Verification items for the finished model (mm, model axes). A direction names the side the tool comes from. Coordinates: 2 decimals unless noted, no trailing zeros. Write each loop counter-clockwise with the first axis right and the second up, starting at its lowest first coordinate (ties: lowest second). Pieces come first, ordered by that corner, then holes. Notation, with made-up numbers: (-17.75, 23.5) - (-2.75, 23.5) arc R22 cw to (-2.75, 59.5) - close; hole circle Ø8 at (-25, 10). An arc over 180 degrees is marked (long way). Use one line per item in the form item = value. Start each with the question number.
(1) Material ranges on line 1 (Y direction, x = -1, z = -2); line 2 (Y direction, x = 2, z = 1.75); line 3 (Y direction, x = -3.5, z = 4), recorded low to high. Write a range as [from, to].
(2) Gauge pin test, flat ends, axial feed: pin 1 Ø1 at (x, z) = (1.5, -3) entering from +Y; pin 2 Ø6 at (x, y) = (-3.5, 3) entering from +Z; pin 3 Ø3 at (y, z) = (8.5, -0.5) entering from -X; pin 4 Ø3 at (y, z) = (12, -4.5) entering from +X. Record the tip position at first contact, or that the pin passes through.
(3) Sectioned sample at D-D (y = 8.25). Record the cut outline in (x, z).
(4) Sectioned sample at C-C (y = 2). Record the cut outline in (x, z), and give its area (3 significant figures).
(5) Tool access check on faces 1 (the flat face through (-1.8, 5.6, 3)), 2 (the flat face through (-3.5, 6, 0)), 3 (the flat face through (3.5, 6, 0)). Record the directions out of +Z, -Z, +X, -X, +Y, -Y that give a thin tool (end or side, any length) a straight path to the whole face; none if there is none.
(6) Sectioned sample at B-B (z = 0). Record the cut outline in (x, y).
(7) Sectioned sample at A-A (y = 5.75). Record the cut outline in (x, z).
Autodesk Fusion 360 part; units mm, degrees
sketch "Sketch1" plane through (0, 0, 0) normal (0, 1, 0) x (1, 0, 0)
  circle A0 centre (0, 0) radius 6
  dimension "d1" = 12
extrude "Extrude1" add sketch "Sketch1" along normal blind 3 makes body 1
chamfer "Chamfer1" distance 0.5 angle 45 2 edges at (-5.594, 3, 2.1697) (-5.594, 0, 2.1697) on bodies 1
sketch "Sketch2" plane through (0, 3, 0) normal (0, 1, 0) x (-1, 0, 0)
  circle A0 centre (0, 0) radius 5.5
  line L0 (-3.5, -2.0207) -> (0, -4.0415)
  line L1 (0, -4.0415) -> (3.5, -2.0207)
  line L2 (3.5, -2.0207) -> (3.5, 2.0207)
  line L3 (3.5, 2.0207) -> (0, 4.0415)
  line L4 (0, 4.0415) -> (-3.5, 2.0207)
  line L5 (-3.5, 2.0207) -> (-3.5, -2.0207)
extrude "Extrude2" add sketch "Sketch2" along normal blind 5 contours L0 L1 L2 L3 L4 L5 bodies 1
ref_plane "WorkPlane1" through (0, 10, 0) normal (0, 1, 0) x (0, 0, 1)
sketch "Sketch3" plane through (0, 10, 0) normal (0, 1, 0) x (1, 0, 0)
  circle A0 centre (0, 0) radius 2.5
  dimension "d8" = 5
extrude "Extrude3" add sketch "Sketch3" along normal blind 5 separate body makes body 2
sketch "Sketch4" plane through (0, 0, 0) normal (0, 0, 1) x (1, 0, 0)
  arc A0 (-2.5, 8) -> (-2.5, 10) centre (-3.25, 9) ccw
  line L0 (-2.5, 10) -> (0, 10)
  line L1 (0, 10) -> (0, 8)
  line L2 (0, 8) -> (-2.5, 8)
revolve "Revolve1" add sketch "Sketch4" angle 360 about axis through (0, 10, 0) along (0, -1, 0) bodies 1 2
chamfer "Chamfer2" distance 0.25 angle 45 1 edges at (-2.3308, 15, 0.904) on bodies 1
thread "Thread1" thread offset 0 thread length 10
fillet "Fillet1" radius 0.25 6 edges at (1.75, 3, 3.0311) (3.5, 3, 0) (1.75, 3, -3.0311) (-1.75, 3, -3.0311) (-3.5, 3, 0) (-1.75, 3, 3.0311) on bodies 1
Answers below:
q1.line_1 = [0, 8.27], [9.73, 15]
q1.line_2 = [0, 8]
q1.line_3 = [0, 3]
q2.pin_1 = 8
q2.pin_2 = 5.98
q2.pin_3 = -3.5
q2.pin_4 = through
q3.outline = circle Ø4.5 at (0, 0)
q4.outline = circle Ø12 at (0, 0)
q4.area = 113 mm2
q5.face_1 = +Z, -X, +Y
q5.face_2 = +Z, -Z, -X, +Y
q5.face_3 = +Z, -Z, +X, +Y
q6.outline = (-6, 0.5) - (-5.5, 0) - (5.5, 0) - (6, 0.5) - (6, 2.5) - (5.5, 3) - (3.75, 3) arc R0.25 cw to (3.5, 3.25) - (3.5, 8) - (2.5, 8) arc R1.25 cw to (2.5, 10) - (2.5, 14.75) - (2.25, 15) - (-2.25, 15) - (-2.5, 14.75) - (-2.5, 10) arc R1.25 cw to (-2.5, 8) - (-3.5, 8) - (-3.5, 3.25) arc R0.25 cw to (-3.75, 3) - (-5.5, 3) - (-6, 2.5) - close
q7.outline = (-3.5, -2.02) - (0, -4.04) - (3.5, -2.02) - (3.5, 2.02) - (0, 4.04) - (-3.5, 2.02) - close
